Model file for the job. Use its own axes, mm. A direction names the side the tool comes from. Round coordinates to 2 decimals unless told otherwise and drop trailing zeros. Order: outer loops, then holes, each group sorted by start corner. A loop starts at its lowest first (then second) coordinate and runs counter-clockwise, first axis right, second up. Notation, with made-up numbers: (-33, 63.5) - (-28, 63.5) arc R23 cw to (-28, 73.5) - close; hole circle Ø6 at (-39.5, 17.25). An arc over 180 degrees is marked (long way). Write item = value, one per line.
Autodesk Inventor part; units mm, degrees
ref_plane "YZ Plane" through (0, 0, 0) normal (1, 0, 0) x (0, 1, 0)
ref_plane "XZ Plane" through (0, 0, 0) normal (0, 1, 0) x (-1, 0, 0)
ref_plane "XY Plane" through (0, 0, 0) normal (0, 0, 1) x (1, 0, 0)
sketch "Sketch1" plane through (0, 0, 0) normal (0, 1, 0) x (-1, 0, 0)
  line L0 (0, 0) -> (67.31, 0)
  line L1 (67.31, 0) -> (67.31, -40.005)
  line L2 (67.31, -40.005) -> (0, -40.005)
  line L3 (0, -40.005) -> (0, 0)
  dimension "d0" = 40.005
  dimension "d1" = 67.31
extrude "Extrusion1" add sketch "Sketch1" along normal blind 3.175
sketch "Sketch2" plane through (0, 3.175, 0) normal (0, 1, 0) x (1, 0, 0)
  circle A0 centre (-13.97, 27.305) radius 6.35
  line L0 (0, 0) -> (0, 40.005)
  line L1 (-67.31, 0) -> (0, 0)
  line L2 (0, 40.005) -> (-67.31, 40.005)
  circle A1 centre (-5.08, 6.35) radius 1.5875
  circle A2 centre (-22.68, 6.35) radius 1.5875
  dimension "d4" = 13.97
  dimension "d28" = 12.7
  dimension "d29" = 12.7
  dimension "d30" = 3.175
  dimension "d31" = 3.175
  dimension "d32" = 5.08
  dimension "d33" = 17.6
  dimension "d34" = 6.35
  dimension "d35" = 6.35
extrude "Extrusion2" cut sketch "Sketch2" against normal blind 6.35
sketch "Sketch3" plane through (0, 0, 0) normal (0, -1, 0) x (1, 0, 0)
  line L0 (0, -40.005) -> (-67.31, -40.005)
  line L1 (-67.31, 0) -> (0, 0)
  line L2 (-67.31, -40.005) -> (-51.435, -40.005)
  line L3 (-51.435, -40.005) -> (-51.435, 0)
  line L4 (-51.435, 0) -> (-67.31, 0)
  line L5 (-67.31, 0) -> (-67.31, -40.005)
  point P0 (-67.31, 0)
  dimension "d8" = 15.875
extrude "Extrusion3" add sketch "Sketch3" along normal blind 16.51
sketch "Sketch4" plane through (-67.31, 3.175, -40.005) normal (-1, 0, 0) x (0, 0, 1)
  line L0 (40.005, -19.685) -> (0, -19.685)
  circle A0 centre (20.0025, -19.685) radius 6.35
  point P0 (40.005, -3.175)
  point P1 (13.6525, -19.685)
  point P2 (26.3525, -19.685)
  dimension "d11" = 12.7
extrude "Extrusion4" cut sketch "Sketch4" against normal blind 6.35 contours L0 A0 picked at (22.0577, -19.1784)
sketch "Sketch5" plane through (-60.96, 3.175, -40.005) normal (-1, 0, 0) x (0, 0, 1)
  line L0 (26.3525, -19.685) -> (13.6525, -19.685)
  line L1 (20.0025, -19.685) -> (20.0025, -3.683)
  circle A0 centre (20.0025, -3.683) radius 3.175
  arc A1 (26.3525, -19.685) -> (13.6525, -19.685) centre (20.0025, -19.685) ccw
  line L2 (24.765, -15.4849) -> (15.24, -15.4849)
  line L3 (24.765, -15.4849) -> (23.1501, -3.267)
  line L4 (15.24, -15.4849) -> (16.8549, -3.267)
  point P0 (40.005, -3.175)
  dimension "d14" = 16.002
  dimension "d15" = 6.35
  dimension "d16" = 9.525
extrude "Extrusion5" cut sketch "Sketch5" along normal blind 2.54 contours A1 L1 A0 L3 | A1 L4 A0 L1 | A0
sketch "Sketch6" plane through (0, 3.175, 0) normal (0, 1, 0) x (1, 0, 0)
  circle A0 centre (-55.88, 28.575) radius 2.1828
  circle A1 centre (-55.88, 9.525) radius 2.1828
  line L0 (-67.31, 40.005) -> (-67.31, 0)
  line L1 (-67.31, 0) -> (0, 0)
  dimension "d19" = 4.3656
  dimension "d20" = 4.3656
  dimension "d21" = 11.43
  dimension "d22" = 11.43
  dimension "d23" = 19.05
  dimension "d24" = 9.525
extrude "Extrusion6" cut sketch "Sketch6" against normal blind 25.4
fillet "Fillet1" radius 1.27 9 edges at (0, 0, -20.0025) (-25.7175, 0, 0) (-25.7175, 0, -40.005) (-51.435, -8.255, 0) (0, 1.5875, 0) (0, 1.5875, -40.005) (-67.31, -6.6675, -40.005) (-51.435, -8.255, -40.005) (-67.31, -6.6675, 0)
sketch "Sketch7" plane through (-67.31, -16.51, -20.0025) normal (-1, 0, 0) x (0, 0, 1)
  line L0 (-18.7325, 0) -> (18.7325, 0)
  circle A0 centre (0, 0) radius 4.7625
  point P0 (20.0025, 16.51)
  point P1 (4.7625, 0)
  point P2 (-4.7625, 0)
  dimension "d38" = 9.525
extrude "Extrusion7" cut sketch "Sketch7" against normal blind 25.4 contours A0 L0 picked at (1.1883, 1.0527)
properties part number "SwerveDriveBracket_B"
1) Cut at B-B (z = -6.35). Write the cut outline in (x, y) (1 decimal).
Conclusion:
outline = (-67.3, -16.5) - (-51.4, -16.5) - (-51.4, 0) - (-24.3, 0) - (-24.3, 3.2) - (-67.3, 3.2) - close; (-21.1, 0) - (-6.7, 0) - (-6.7, 3.2) - (-21.1, 3.2) - close; (-3.5, 0) - (-1.3, 0) arc R1.3 ccw to (0, 1.3) - (0, 3.2) - (-3.5, 3.2) - close
2) Wall check: line 1 along X through (y, z) = (2.3, -6.35); line 2 along Z through (x, y) = (-55.88, -9.5) (3 decimals); line 3 along X through (y, z) = (-4.25, -28.5) (3 decimals). Give the ranges that are in metal, low to high.
Conclusion:
line_1 = -67.31 to -24.27, -21.09 to -6.67, -3.49 to 0
line_2 = -40.005 to -30.758, -26.392 to -11.708, -7.342 to 0
line_3 = -67.31 to -58.062, -53.698 to -51.435
3) Cut at D-D (y = 2). Give the number of separate pieces and of enclosed holes in the cut face, and give its area (3 significant figures).
Conclusion:
separate_pieces = 1
enclosed_holes = 6
area = 2,510 mm^2
4) Cut at C-C (x = -13.97). Write the cut outline in (y, z) (3 decimals).
Conclusion:
outline = (0, -38.735) arc R1.27 ccw to (1.27, -40.005) - (3.175, -40.005) - (3.175, -33.655) - (0, -33.655) - close; (0, -20.955) - (3.175, -20.955) - (3.175, 0) - (1.27, 0) arc R1.27 ccw to (0, -1.27) - close
5) Cut at A-A (x = -55.88). Write the cut outline in (y, z) (1 decimal), and give its area (3 significant figures).
Conclusion:
outline = (-16.5, -40) - (3.2, -40) - (3.2, -30.8) - (-16.5, -30.8) - close; (-16.5, -26.4) - (3.2, -26.4) - (3.2, -11.7) - (-16.5, -11.7) - (-16.5, -15.2) arc R4.8 cw to (-16.5, -24.8) - close; (-16.5, -7.3) - (3.2, -7.3) - (3.2, 0) - (-16.5, 0) - close
area = 580 mm^2
6) 3-axis set-ups, long thin cutter, end or side, ignore diameter. For faces 1 (the face through (-26, 0, -20)), 2 (the face through (-51.8, -7.74, -0.38)), 3 (the face through (-62.21, -6.29, -23.97)), 4 (the face through (-64.89, -10.16, -19.86)): which of +Z, -Z, +X, -X, +Y, -Y reach the whole face in a straight line?
Conclusion:
face_1 = +Z, -Z, +X, -Y
face_2 = +Z, +X, -Y
face_3 = -Y
face_4 = -X, -Y
7) Mould opens along X. For faces 5 (the face through (-66.93, -6.53, -39.64)), 6 (the face through (-27.348, 0.362, -0.382)), 7 (the face through (-24.266, 1.61, -6.42)) say: +X half, -X half, draft (parallel to the pull), parting line (faces both ways), or undercut.
Conclusion:
face_5 = -X half
face_6 = draft
face_7 = undercut
8) Flat gauge pins, fed straight in: pin 1 Ø8 at (y, z) = (0.5, -14) entering from +X; pin 2 Ø8.5 at (y, z) = (-7.5, -23.5) entering from +X (3 decimals); pin 3 Ø11 at (x, z) = (-19.5, -13.5) entering from -Y. Where does each tip first touch, or does it go through?
Conclusion:
pin_1 = 0
pin_2 = -51.435
pin_3 = 0
